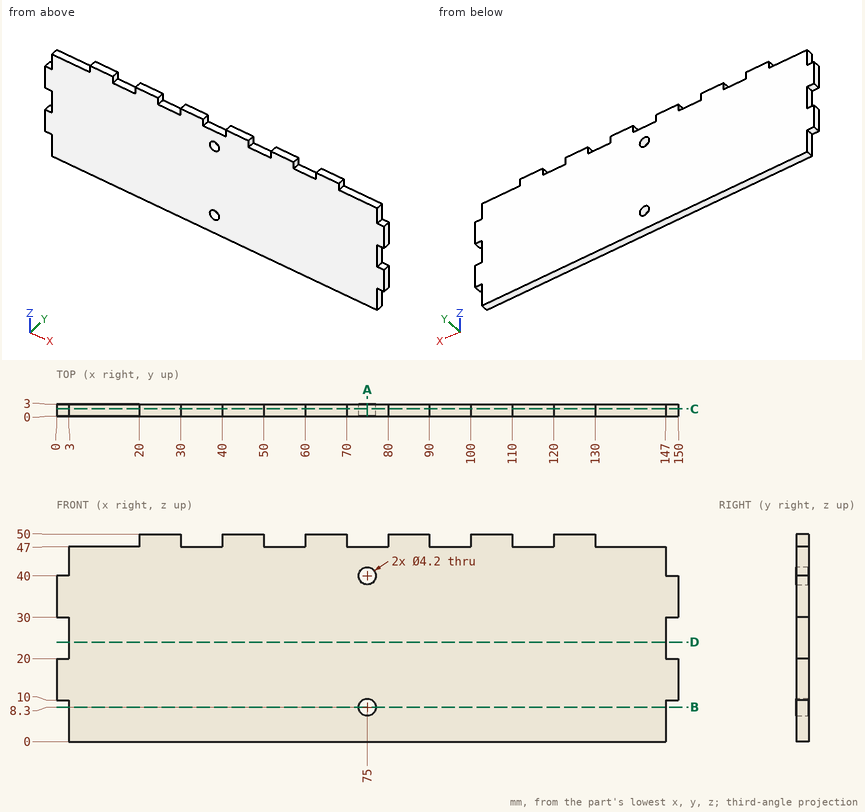
Study the drawing (mm; zero at the part's minimum x, y, z) and answer. Round coordinates to 2 decimals unless told otherwise and drop trailing zeros. Write each loop counter-clockwise with the first axis right and the second up, starting at its lowest first coordinate (ties: lowest second). Pieces come first, ordered by that corner, then holes. Notation, with made-up numbers: (70, 72.25) - (128, 72.25) arc R18 ccw to (128, 95.25) - close; hole circle Ø8 at (-36.5, 14). An arc over 180 degrees is marked (long way). Use a Markdown table: item, result. Add a question column.
1. The part is cut by section A-A (x = 75). Write down the section's boundary in (y, z), and give its area (3 significant figures).
2. Flat-ended cylindrical pins translate along their axes: P1, Ø0.9, axis at y = 1, z = 48, coming from the +X side; P2, Ø1.5, axis at y = 1, z = 42, coming from the -X side; P3, Ø1.5, axis at x = 148, y = 1.5, coming from the +Z side. Find the tip coordinate at first contact, or state that the pin passes through.
3. Consider line 1 (Z direction, x = 116.5, y = 2.6); line 2 (X direction, y = 2.2, z = 46); line 3 (X direction, y = 2.75, z = 38.5). Determine where each line is inside the solid, lowest interval first.
4. The part is cut by section C-C (y = 1.85). Give the number of separate pieces and of enclosed holes in the cut face, and give its area (3 significant figures).
5. The part is cut by section B-B (z = 8.3). Write down the section's boundary in (x, y), and give its area (3 significant figures).
6. The part is cut by section D-D (z = 24). Write down the section's boundary in (x, y), and give its area (3 significant figures).
Reported:
| question | item | result |
|---|---|---|
| 1 | outline | (0, 0) - (3, 0) - (3, 6.2) - (0, 6.2) - close; (0, 10.4) - (3, 10.4) - (3, 37.9) - (0, 37.9) - close; (0, 42.1) - (3, 42.1) - (3, 47) - (0, 47) - close |
| 1 | area | 116 mm^2 |
| 2 | P1 | x = 130 |
| 2 | P2 | x = 3 |
| 2 | P3 | z = 40 |
| 3 | line 1 | 0 to 47 |
| 3 | line 2 | 3 to 147 |
| 3 | line 3 | 0 to 73.53, 76.47 to 150 |
| 4 | separate pieces | 1 |
| 4 | enclosed holes | 2 |
| 4 | area | 7,040 mm^2 |
| 5 | outline | (3, 0) - (72.9, 0) - (72.9, 3) - (3, 3) - close; (77.1, 0) - (147, 0) - (147, 3) - (77.1, 3) - close |
| 5 | area | 419 mm^2 |
| 6 | outline | (3, 0) - (147, 0) - (147, 3) - (3, 3) - close |
| 6 | area | 432 mm^2 |
